Work out the finished part from the listing and answer in its coordinate system (mm). A direction names the side the tool comes from. Round coordinates to 2 decimals unless told otherwise and drop trailing zeros. Order: outer loops, then holes, each group sorted by start corner. A loop starts at its lowest first (then second) coordinate and runs counter-clockwise, first axis right, second up. Notation, with made-up numbers: (78, -31.75) - (136, -31.75) arc R19 ccw to (136, -16.75) - close; hole circle Ø2 at (-29.75, -39). An arc over 180 degrees is marked (long way). Answer in a Markdown table with one row per item.
Autodesk Inventor part; units mm, degrees
ref_plane "Płaszczyzna konstrukcyjna3" through (0, 12, 0) normal (0, 1, 0) x (-1, 0, 0)
ref_plane "YZ Plane" through (0, 0, 0) normal (1, 0, 0) x (0, 1, 0)
ref_plane "XY Plane" through (0, 0, 0) normal (0, 0, 1) x (1, 0, 0)
sketch "Szkic1" plane through (0, 0, 0) normal (0, 1, 0) x (-1, 0, 0)
  line L0 (57.6, -28.8) -> (-57.6, -28.8)
  line L1 (-57.6, -28.8) -> (-57.6, 28.8)
  line L2 (-57.6, 28.8) -> (57.6, 28.8)
  line L3 (57.6, 28.8) -> (57.6, -28.8)
  line L4 (57.6, -28.8) -> (-57.6, 28.8) construction
  line L5 (-57.6, -28.8) -> (57.6, 28.8) construction
  point P0 (0, 0)
  dimension "d0" = 115.2
  dimension "d1" = 57.6
ref_plane "Płaszczyzna konstrukcyjna3" through (0, 12, 0) normal (0, 1, 0) x (-1, 0, 0)
sketch "Szkic11" plane through (0, 12, 0) normal (0, 1, 0) x (-1, 0, 0)
  line L0 (-5, -12.5) -> (5, -12.5)
  line L1 (5, -12.5) -> (5, 12.5)
  line L2 (5, 12.5) -> (-5, 12.5)
  line L3 (-5, 12.5) -> (-5, -12.5)
  line L4 (-5, -12.5) -> (5, 12.5) construction
  line L5 (5, -12.5) -> (-5, 12.5) construction
  point P0 (0, 0)
  dimension "d41" = 10
  dimension "d42" = 25
loft "Wyciągnięcie złożone3" add profiles "Szkic11", "Szkic1"
shell "Skorupa3" thickness 1.2 removed faces 1 at (-19.2, 0, 9.6)
sketch "Szkic12" plane through (-4.8649, 10.8, -12.1059) normal (0, -1, 0) x (1, 0, 0)
  line L0 (0, 0) -> (0, 24.2118)
  line L1 (9.7297, 0) -> (57.0697, -14.67)
  line L2 (0, 24.2118) -> (9.7297, 24.2118)
  line L3 (9.7297, 24.2118) -> (9.7297, 0)
  line L4 (9.7297, 0) -> (0, 0)
  line L5 (0, 0) -> (0, 24.2118)
  point P0 (4.8649, 12.1059)
extrude "Wyciągnięcie proste7" cut sketch "Szkic12" against normal blind 10
sketch "Szkic13" plane through (-57.6, 0, -28.8) normal (0, -1, 0) x (1, 0, 0)
  line L0 (115.2, 57.6) -> (115.2, 0)
  line L1 (52.6, 16.3) -> (0, 0)
  line L2 (115.2, 57.6) -> (0, 57.6)
  line L3 (0, 57.6) -> (0, 0)
  line L4 (0, 0) -> (115.2, 0)
  line L5 (115.2, 0) -> (115.2, 57.6)
  line L6 (5.3951, 55.5759) -> (109.8049, 55.5759)
  line L7 (109.8049, 2.0241) -> (5.3951, 2.0241)
  line L8 (109.8049, 55.5759) -> (5.3951, 55.5759)
  line L9 (5.3951, 55.5759) -> (5.3951, 2.0241)
  line L10 (5.3951, 2.0241) -> (109.8049, 2.0241)
  line L11 (109.8049, 2.0241) -> (109.8049, 55.5759)
  point P0 (57.6, 28.8)
extrude "Wyciągnięcie proste8" add sketch "Szkic13" along normal blind 8
sketch "Szkic14" plane through (-57.6, -8, -28.8) normal (0, -1, 0) x (1, 0, 0)
  line L0 (115.2, 57.6) -> (0, 57.6)
  line L1 (115.2, 0) -> (0, 0)
  line L2 (0, 0) -> (0, 57.6)
  line L3 (0, 57.6) -> (115.2, 57.6)
  line L4 (115.2, 57.6) -> (115.2, 0)
  line L5 (115.2, 0) -> (0, 57.6) construction
  line L6 (0, 0) -> (115.2, 57.6) construction
  line L7 (116.4, 0) -> (-1.2, 0)
  line L8 (-1.2, 0) -> (-1.2, 57.6)
  line L9 (-1.2, 57.6) -> (116.4, 57.6)
  line L10 (116.4, 57.6) -> (116.4, 0)
  line L11 (116.4, 0) -> (-1.2, 57.6) construction
  line L12 (-1.2, 0) -> (116.4, 57.6) construction
  point P0 (57.6, 28.8)
  dimension "d52" = 117.6
extrude "Wyciągnięcie proste9" add sketch "Szkic14" against normal blind 4 contours L9 L10 L7 L4 | L2 L7 L8 L9
sketch "Szkic15" plane through (-5, 12, -12.5) normal (0, 1, 0) x (1, 0, 0)
  line L0 (9.8649, -24.6059) -> (9.8649, -0.3941)
  line L1 (0.1351, -13.1) -> (9.8649, -13.1)
  line L2 (9.8649, -13.1) -> (9.8649, -11.9)
  line L3 (9.8649, -11.9) -> (0.1351, -11.9)
  line L4 (0.1351, -11.9) -> (0.1351, -13.1)
  line L5 (0.1351, -13.1) -> (9.8649, -11.9) construction
  line L6 (9.8649, -13.1) -> (0.1351, -11.9) construction
  point P0 (5, -12.5)
  dimension "d55" = 1.2
extrude "Wyciągnięcie proste10" add sketch "Szkic15" against normal blind 1.2
pattern_linear "Szyk prostokątny3" count 2 spacing 6 along (0, 0, -1) of "Wyciągnięcie proste10"
pattern_linear "Szyk prostokątny4" count 2 spacing 6 along (0, 0, 1) of "Wyciągnięcie proste10"
properties part number "lejek"
1) Which of the six approach directions +Z, -Z, +X, -X, +Y, -Y give full straight-line access (tool end or side, diameter ignored) to faces 1 (the face through (58.8, -6, 0)), 2 (the face through (1, -4, -26.776)), 3 (the face through (-57.6, -2, 0))?
Filled in:
| item | result |
|---|---|
| face 1 | +Z, -Z, +X, +Y, -Y |
| face 2 | -Y |
| face 3 | +Z, -Z, -X, +Y |
2) Each of these flat-tipped pins is pushed along its axis until it touches: pin 1 (3 mm diameter, centred on x = 28, z = 7, fed in from -Y); pin 2 (1.3 mm diameter, centred on x = 2, y = 11.5, fed in from -Z); pin 3 (0.6 mm diameter, centred on x = 1.5, z = -6, fed in from -Y); pin 4 (10 mm diameter, centred on x = 2.5, z = 14, fed in from +Y). Where does it stop, or does it pass through?
Filled in:
| item | result |
|---|---|
| pin 1 | stops at y = 5.18 |
| pin 2 | stops at z = -14.06 |
| pin 3 | stops at y = 10.8 |
| pin 4 | stops at y = 12 |
3) Find section B-B, the plane y = -6.5. Give the vertices of the cut face in (x, z).
Filled in:
| item | result |
|---|---|
| outline | (-58.8, -28.8) - (58.8, -28.8) - (58.8, 28.8) - (-58.8, 28.8) - close; hole (-52.2, -26.78) - (52.2, -26.78) - (52.2, 26.78) - (-52.2, 26.78) - close |
4) Find section A-A, the plane y = -1.25. Give the vertices of the cut face in (x, z).
Filled in:
| item | result |
|---|---|
| outline | (-57.6, -28.8) - (57.6, -28.8) - (57.6, 28.8) - (-57.6, 28.8) - close; hole (-52.2, -26.78) - (52.2, -26.78) - (52.2, 26.78) - (-52.2, 26.78) - close |
5) The mould has two halves that part along X. Classify faces 4 (the face through (0, 12, 0)), 5 (the face through (-52.205, -4, 0)), 6 (the face through (57.6, -2, 0)), 7 (the face through (-1, -4, 26.776)): released by +X, released by -X, zero draft, split by the parting line, or undercut.
Filled in:
| item | result |
|---|---|
| face 4 | zero draft |
| face 5 | undercut |
| face 6 | released by +X |
| face 7 | undercut |
6) Find the intervals of material crossed by probe 1 along Z at (x, y) = (-14, -1.5); probe 2 along X at (y, z) = (-5, -1); probe 3 along X at (y, z) = (-2.5, 19), in increasing order. Write a range as from..to.
Filled in:
| item | result |
|---|---|
| probe 1 | z = -28.8..-26.78, 26.78..28.8 |
| probe 2 | x = -58.8..-52.2, 52.2..58.8 |
| probe 3 | x = -57.6..-52.2, 52.2..57.6 |
